from build123d import *

# Parameters (mm, degrees)
SKETCH1_R           = 35
SKETCH1_R_2         = 23.425
SKETCH1_R_3         = 1.975
BOSS_EXTRUDE1_DEPTH = 5
SKETCH4_R           = 35
SKETCH4_R_2         = 23.425
SKETCH4_R_3         = 1.975
BOSS_EXTRUDE3_DEPTH = 2


with BuildPart() as part:
    # Sketch1 → Boss-Extrude1 (new body)
    with BuildSketch(Plane.XY):
        Circle(SKETCH1_R)
        Circle(SKETCH1_R_2, mode=Mode.SUBTRACT)
        with Locations((0, 29)):
            Circle(SKETCH1_R_3, mode=Mode.SUBTRACT)
        with Locations((29, 0)):
            Circle(SKETCH1_R_3, mode=Mode.SUBTRACT)
        with Locations((0, -29)):
            Circle(SKETCH1_R_3, mode=Mode.SUBTRACT)
        with Locations((-29, 0)):
            Circle(SKETCH1_R_3, mode=Mode.SUBTRACT)
    extrude(amount=BOSS_EXTRUDE1_DEPTH)

    # Sketch4 → Boss-Extrude3 (add)
    with BuildSketch(Plane.XY.offset(5)):
        Circle(SKETCH4_R)
        Circle(SKETCH4_R_2, mode=Mode.SUBTRACT)
        with Locations((0, 29)):
            Circle(SKETCH4_R_3, mode=Mode.SUBTRACT)
        with Locations((29, 0)):
            Circle(SKETCH4_R_3, mode=Mode.SUBTRACT)
        with Locations((0, -29)):
            Circle(SKETCH4_R_3, mode=Mode.SUBTRACT)
        with Locations((-29, 0)):
            Circle(SKETCH4_R_3, mode=Mode.SUBTRACT)
    extrude(amount=BOSS_EXTRUDE3_DEPTH)


solid = part.part
Model file for the job. Use its own axes, mm. Give positions to 0.01 mm unless a question says otherwise; leave off trailing zeros. Write each loop counter-clockwise with the first axis right and the second up, starting at its lowest first coordinate (ties: lowest second). Pieces come first, ordered by that corner, then holes. Notation, with made-up numbers: M 87,4 L 97,4 A22 cw 97,29 Z; hole C 49.25,61.5 d3. An arc over 180 degrees is marked long. One line per item, written item: value. Start each with the question number.
Q1. Saw through at D-D, the plane y = 17. Write the cut outline in (x, z), plus the area to 3 significant figures.
Q2. Probe probe 1 along Y at (x, z) = (0, 2) (3 decimals); probe 2 along Y at (x, z) = (-1.5, 5); probe 3 along Y at (x, z) = (12, 1.25). List the from-to ranges inside material, lowest first. Write a range as [from, to].
Q3. Saw through at C-C, the plane x = 29. Write the cut outline in (y, z) (3 decimals), plus the area to 3 significant figures.
Q4. Two-plate mould, pull along X, no slides. Class faces 1 (the flat face through (-24, 0, 0)), 2 (the cylindrical face through (-28, -21, 3)), 3 (the cylindrical face through (-1.57, -30.2, 3.45)): +X half, -X half, draft (parallel to the pull), parting line (faces both ways), or undercut.
Q5. Saw through at B-B, the plane z = 4. Write the cut outline in (x, y) (3 decimals).
Q6. Saw through at A-A, the plane y = 0. Write the cut outline in (x, z) (3 decimals), plus the area to 3 significant figures.
Q7. Drop flat-ended pins along their axis: pin 1 Ø2 at (x, z) = (27, 3) entering from +Y; pin 2 Ø2 at (x, z) = (14, 6) entering from -Y; pin 3 Ø1 at (x, z) = (-9, 4) entering from +Y. Give the stop position or say it passes through.
Output values:
1. outline: M -30.59,0 L -16.12,0 L -16.12,7 L -30.59,7 Z; M 16.12,0 L 30.59,0 L 30.59,7 L 16.12,7 Z
1. area: 203 mm²
2. probe 1: y = [-35, -30.975], [-27.025, -23.425], [23.425, 27.025], [30.975, 35]
2. probe 2: y = [-34.97, -30.28], [-27.72, -23.38], [23.38, 27.72], [30.28, 34.97]
2. probe 3: y = [-32.88, -20.12], [20.12, 32.88]
3. outline: M -19.596,0 L -1.975,0 L -1.975,7 L -19.596,7 Z; M 1.975,0 L 19.596,0 L 19.596,7 L 1.975,7 Z
3. area: 247 mm²
4. face 1: draft
4. face 2: parting line
4. face 3: undercut
5. outline: C 0,0 d70; hole C -29,0 d3.95; hole C 0,0 d46.85; hole C 0,-29 d3.95; hole C 0,29 d3.95; hole C 29,0 d3.95
6. outline: M -35,0 L -30.975,0 L -30.975,7 L -35,7 Z; M -27.025,0 L -23.425,0 L -23.425,7 L -27.025,7 Z; M 23.425,0 L 27.025,0 L 27.025,7 L 23.425,7 Z; M 30.975,0 L 35,0 L 35,7 L 30.975,7 Z
6. area: 107 mm²
7. pin 1: stops at y = 23.43
7. pin 2: stops at y = -32.5
7. pin 3: stops at y = 33.95
